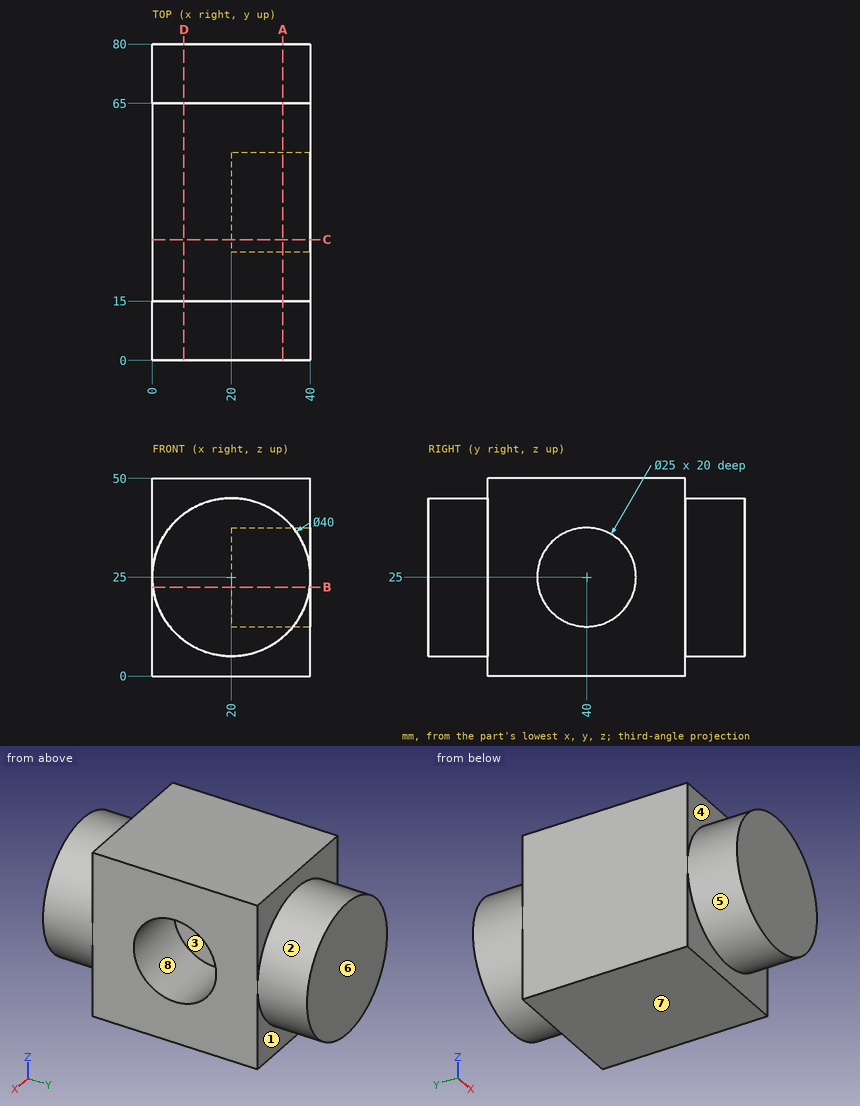
Can you work these out from the drawing? Everything is in mm from the part's minimum corner. A direction names the side the tool comes from. Round coordinates to 2 decimals unless told otherwise and drop trailing zeros. Loops run counter-clockwise (first coordinate to the right, second up) from the corner with the lowest first, then second, coordinate; pieces in that order, holes last. Notation, with made-up numbers: (51.5, 26.25) -> (105.5, 26.25) arc R6 cw to (105.5, 35.25) -> close; hole circle Ø2 at (5, 27.5). An arc over 180 degrees is marked (long way). Answer in a Markdown table with one row per item.
Item 1: Suppose I cut it at A-A, the plane x = 33. List the corners of the cut face in (y, z) for me.
Answer block:
| item | result |
|---|---|
| outline | (0, 9.8) -> (15, 9.8) -> (15, 0) -> (65, 0) -> (65, 9.8) -> (80, 9.8) -> (80, 40.2) -> (65, 40.2) -> (65, 50) -> (15, 50) -> (15, 40.2) -> (0, 40.2) -> close; hole circle Ø25 at (40, 25) |
Item 2: Suppose I cut it at D-D, the plane x = 8. List the corners of the cut face in (y, z) for me.
Answer block:
| item | result |
|---|---|
| outline | (0, 9) -> (15, 9) -> (15, 0) -> (65, 0) -> (65, 9) -> (80, 9) -> (80, 41) -> (65, 41) -> (65, 50) -> (15, 50) -> (15, 41) -> (0, 41) -> close |
Item 3: Suppose I cut it at B-B, the plane z = 22.5. List the corners of the cut face in (x, y) for me.
Answer block:
| item | result |
|---|---|
| outline | (0, 15) -> (0.16, 15) -> (0.16, 0) -> (39.84, 0) -> (39.84, 15) -> (40, 15) -> (40, 27.75) -> (20, 27.75) -> (20, 52.25) -> (40, 52.25) -> (40, 65) -> (39.84, 65) -> (39.84, 80) -> (0.16, 80) -> (0.16, 65) -> (0, 65) -> close |
Item 4: We'd pull the mould along Z, two halves only. Please class the marked faces 6, 7 and 8: released by +Z, released by -Z, zero draft, split by the parting line, or undercut.
Answer block:
| item | result |
|---|---|
| face 6 | zero draft |
| face 7 | released by -Z |
| face 8 | undercut |
Item 5: Suppose I cut it at C-C, the plane y = 30.5. List the corners of the cut face in (x, z) for me.
Answer block:
| item | result |
|---|---|
| outline | (0, 0) -> (40, 0) -> (40, 16.88) -> (20, 16.88) -> (20, 33.12) -> (40, 33.12) -> (40, 50) -> (0, 50) -> close |
Item 6: On a 3-axis mill with a long thin cutter (end or side, diameter ignored), from which of +Z, -Z, +X, -X, +Y, -Y can I reach the whole of each face in a straight line? I mean the marked faces 1, 2, 3, 4 and 5. Say none if no direction works.
Answer block:
| item | result |
|---|---|
| face 1 | -Z, +Y |
| face 2 | +Y |
| face 3 | +X |
| face 4 | +Z, -Y |
| face 5 | -Y |
Item 7: If I drill on probe 1 along Z at (x, y) = (27, 40); probe 2 along X at (y, z) = (32, 17.5); probe 3 along Y at (x, z) = (21.5, 18), over which ranges is the centre line in solid material (lowest first)?
Answer block:
| item | result |
|---|---|
| probe 1 | 0 to 12.5, 37.5 to 50 |
| probe 2 | 0 to 20 |
| probe 3 | 0 to 29.64, 50.36 to 80 |
Item 8: Will these pins go through, and if not, where does the flat tip stop? P1, Ø2, axis at x = 33.5, y = 68, coming from the +Z side; P2, Ø8, axis at x = 8.5, y = 69.5, coming from the +Z side; P3, Ø2, axis at x = 6, z = 5, coming from the +Y side.
Answer block:
| item | result |
|---|---|
| P1 | z = 40.61 |
| P2 | z = 43.54 |
| P3 | y = 65 |
